Geometry: final body of the model. Coordinates: model frame, mm. A direction names the side the tool comes from. Round coordinates to 2 decimals unless told otherwise and drop trailing zeros. Write each loop counter-clockwise with the first axis right and the second up, starting at its lowest first coordinate (ties: lowest second). Pieces come first, ordered by that corner, then holes. Notation, with made-up numbers: (83.25, 87.25) -> (106.25, 87.25) arc R22 cw to (106.25, 108.25) -> close; hole circle Ø9 at (-10.75, 34.25). An arc over 180 degrees is marked (long way). Use one line per item in the form item = value. Start each with the question number.
1. Cut plane A-A, the plane y = 6.5. Return the cut outline in (x, z), plus the area to 3 significant figures.
2. Line query: L1, parallel to Y at x = -8, z = 3; L2, parallel to Y at x = -6.75, z = 5; L3, parallel to Z at x = -9.75, y = 11. Output: solid intervals per line, ascending.
3. Cut plane D-D, the plane y = 3.5. Return the cut outline in (x, z).
4. Reachability of faces 1 (the face through (-8, 14, 0)), 2 (the face through (-6, 4, 9)) from +Z, -Z, +X, -X, +Y, -Y: full face, straight path, thin tool, end or side. Return the list, or none.
5. Cut plane B-B, the plane x = -5.75. Return the cut outline in (y, z), plus the area to 3 significant figures.
6. Draft query along Y for faces 3 (the face through (-8, 0, 4)), 4 (the face through (-8, 29, 8)), 5 (the face through (-8, 14, 16)), 6 (the face through (-9.5, 3.57, 12.55)). Return one class per face: pulls with the +Y half, pulls with the -Y half, needs draft (parallel to the pull), parting line crosses it, or undercut.
7. Pin query (flat end, axial travel): pin 1 Ø4 at (y, z) = (11, 8) entering from -X. Return the tip coordinate at first contact, or that it passes through.
8. Cut plane C-C, the plane z = 8. Return the cut outline in (x, y), plus the area to 3 significant figures.
Autodesk Inventor part; units mm, degrees
ref_plane "YZ Plane" through (0, 0, 0) normal (1, 0, 0) x (0, 1, 0)
ref_plane "XZ Plane" through (0, 0, 0) normal (0, 1, 0) x (-1, 0, 0)
ref_plane "XY Plane" through (0, 0, 0) normal (0, 0, 1) x (1, 0, 0)
sketch "Sketch1" plane through (0, 0, 0) normal (0, 1, 0) x (-1, 0, 0)
  line L0 (0, 0) -> (16, 0)
  line L1 (16, 0) -> (16, 16)
  line L2 (16, 16) -> (0, 16)
  line L3 (0, 16) -> (0, 0)
  dimension "d0" = 16
  dimension "d1" = 16
extrude "Extrusion1" add sketch "Sketch1" along normal blind 29
sketch "Sketch2" plane through (-16, 0, 16) normal (0, 0, 1) x (1, 0, 0)
  circle A0 centre (8, 3.5) radius 1.5
  circle A1 centre (8, 21) radius 4
  dimension "d5" = 3
  dimension "d7" = 8
extrude "Extrusion2" cut sketch "Sketch2" against normal blind 29
sketch "Sketch3" plane through (0, 0, 16) normal (1, 0, 0) x (0, 0, -1)
  line L0 (0, 0) -> (16, 0)
  line L1 (16, 0) -> (16, 29)
  line L2 (0, 0) -> (0, 29)
  line L3 (0, 0) -> (0, 11)
  arc A0 (9, 7.127) -> (7, 7.127) centre (8, 11) ccw
  line L4 (8, 0) -> (9, 0)
  line L5 (9, 0) -> (9, 7.127)
  line L6 (8, 0) -> (7, 0)
  line L7 (7, 0) -> (7, 7.127)
  line L8 (0, 11) -> (4, 11)
  line L9 (12, 11) -> (16, 11)
  dimension "d10" = 11
  dimension "d11" = 8
  dimension "d12" = 1
  dimension "d13" = 1
extrude "Extrusion3" cut sketch "Sketch3" against normal blind 29 contours L7 A0 L5 L0
properties part number "BarClamp_V3" material "Birch"
Outcome:
q1.outline = (-16, 0) -> (0, 0) -> (0, 7) -> (-16, 7) -> close; (-16, 9) -> (0, 9) -> (0, 16) -> (-16, 16) -> close
q1.area = 224 mm^2
q2.L1 = 0 to 2, 5 to 17, 25 to 29
q2.L2 = 0 to 2.67, 4.33 to 8.35, 13.65 to 17.2, 24.8 to 29
q2.L3 = 0 to 4, 12 to 16
q3.outline = (-16, 0) -> (-9.5, 0) -> (-9.5, 7) -> (-16, 7) -> close; (-16, 9) -> (-9.5, 9) -> (-9.5, 16) -> (-16, 16) -> close; (-6.5, 0) -> (0, 0) -> (0, 7) -> (-6.5, 7) -> close; (-6.5, 9) -> (0, 9) -> (0, 16) -> (-6.5, 16) -> close
q4.face_1 = -Z, +X, -X, +Y, -Y
q4.face_2 = +X, -X, -Y
q5.outline = (0, 0) -> (17.69, 0) -> (17.69, 16) -> (0, 16) -> (0, 9) -> (7.13, 9) arc R4 cw (long way) to (7.13, 7) -> (0, 7) -> close; (24.31, 0) -> (29, 0) -> (29, 16) -> (24.31, 16) -> close
q5.area = 294 mm^2
q6.face_3 = pulls with the -Y half
q6.face_4 = pulls with the +Y half
q6.face_5 = needs draft
q6.face_6 = undercut
q7.pin_1 = through
q8.outline = (-16, 15) -> (0, 15) -> (0, 29) -> (-16, 29) -> close; hole circle Ø8 at (-8, 21)
q8.area = 174 mm^2
